```python
from build123d import *

# Parameters (mm, degrees)
F1_DEPTH = 10


with BuildPart() as f1:
    # F0 (on Top) → F1 (new body)
    with BuildSketch(Plane.XY):
        Polygon((2.178894, 24.904867), (0, 25), (0, 29.088151), (-5.051104, 28.646236), (-4.341204, 24.620194), (-6.470476, 24.148146), (-7.528567, 28.096996), (-12.293184, 26.362817), (-10.565457, 22.657695), (-12.5, 21.650635), (-14.544075, 25.191077), (-18.697503, 22.282816), (-16.06969, 19.151111), (-17.67767, 17.67767), (-20.568429, 20.568429), (-23.827618, 16.684278), (-20.478801, 14.339411), (-21.650635, 12.5), (-25.191077, 14.544075), (-27.333921, 9.948733), (-23.492316, 8.550504), (-24.148146, 6.470476), (-28.096996, 7.528567), (-28.977462, 2.535199), (-24.904867, 2.178894), (-25, 0), (-29.088151, 0), (-28.646236, -5.051104), (-24.620194, -4.341204), (-24.148146, -6.470476), (-28.096996, -7.528567), (-26.362817, -12.293184), (-22.657695, -10.565457), (-21.650635, -12.5), (-25.191077, -14.544075), (-22.282816, -18.697503), (-19.151111, -16.06969), (-17.67767, -17.67767), (-20.568429, -20.568429), (-16.684278, -23.827618), (-14.339411, -20.478801), (-12.5, -21.650635), (-14.544075, -25.191077), (-9.948733, -27.333921), (-8.550504, -23.492316), (-6.470476, -24.148146), (-7.528567, -28.096996), (-2.535199, -28.977462), (-2.178894, -24.904867), (0, -25), (0, -29.088151), (5.051104, -28.646236), (4.341204, -24.620194), (6.470476, -24.148146), (7.528567, -28.096996), (12.293184, -26.362817), (10.565457, -22.657695), (12.5, -21.650635), (14.544075, -25.191077), (18.697503, -22.282816), (16.06969, -19.151111), (17.67767, -17.67767), (20.568429, -20.568429), (23.827618, -16.684278), (20.478801, -14.339411), (21.650635, -12.5), (25.191077, -14.544075), (27.333921, -9.948733), (23.492316, -8.550504), (24.148146, -6.470476), (28.096996, -7.528567), (28.977462, -2.535199), (24.904867, -2.178894), (25, 0), (29.088151, 0), (28.646236, 5.051104), (24.620194, 4.341204), (24.148146, 6.470476), (28.096996, 7.528567), (26.362817, 12.293184), (22.657695, 10.565457), (21.650635, 12.5), (25.191077, 14.544075), (22.282816, 18.697503), (19.151111, 16.06969), (17.67767, 17.67767), (20.568429, 20.568429), (16.684278, 23.827618), (14.339411, 20.478801), (12.5, 21.650635), (14.544075, 25.191077), (9.948733, 27.333921), (8.550504, 23.492316), (6.470476, 24.148146), (7.528567, 28.096996), (2.535199, 28.977462), align=None)
    extrude(amount=F1_DEPTH)


solid = f1.part
```
The listing builds one solid part. Answer for the finished solid, in the listing's coordinates (mm). A direction names the side the tool comes from. Coordinates: 2 decimals unless noted, no trailing zeros. Loops run counter-clockwise (first coordinate to the right, second up) from the corner with the lowest first, then second, coordinate; pieces in that order, holes last. Notation, with made-up numbers: M 79,40 L 115,40 A26 ccw 115,64 Z; hole C 63,33 d9. An arc over 180 degrees is marked long. Answer as a JSON object with one key per item and string values. Group by question number.
Item 1: Each of these flat-tipped pins is pushed along its axis until it touches: P1, Ø2, axis at x = 27, z = 7.5, coming from the -Y side; P2, Ø4, axis at x = -5, z = 4, coming from the +Y side; P3, Ø5, axis at x = -4, z = 6.5, coming from the +Y side. Where does it stop, or does it pass through?
Item 2: Which of the six approach directions +Z, -Z, +X, -X, +Y, -Y give full straight-line access (tool end or side, diameter ignored) to faces 1 (the face through (-28.53, 5.07, 4.93)), 2 (the face through (0, 27, 5)), 3 (the face through (-1.1, -24.95, 4.93)), 4 (the face through (25.44, -9.26, 4.93)), 5 (the face through (6.99, 26.09, 4.93))?
Item 3: Determine the mould class of faces 6 (the face through (9.26, 25.44, 4.93)), 7 (the face through (24.95, -1.1, 4.93)), 8 (the face through (6.99, -26.09, 4.93)), 9 (the face through (5.391, -24.387, 4.93)) for opening direction Y: +Y half, -Y half, draft (parallel to the pull), parting line (faces both ways), or undercut.
Item 4: Section B-B (y = -11.5) is taken. Write down the section's boundary in (x, z), and give its area (3 significant figures).
Item 5: Section A-A (y = 13.5) is taken. Write down the section's boundary in (x, z), and give its area (3 significant figures).
Item 6: Consider L1, parallel to X at y = -18.5, z = 8.25; L2, parallel to X at y = 25.5, z = 4.25; L3, parallel to X at y = 26, z = 3.75. Determine where each line is inside the solid, lowest interval first.
Solved:
{
 "1": {"P1": "stops at y = -12.81", "P2": "stops at y = 28.83", "P3": "stops at y = 28.96"},
 "2": {"face 1": "+Z, -Z, -X, +Y", "face 2": "+Z, -Z, +Y", "face 3": "+Z, -Z, -Y", "face 4": "+Z, -Z, +X", "face 5": "+Z, -Z"},
 "3": {"face 6": "+Y half", "face 7": "undercut", "face 8": "-Y half", "face 9": "undercut"},
 "4": {"outline": "M -26.65,0 L -24.66,0 L -24.66,10 L -26.65,10 Z; M -22.17,0 L 26.61,0 L 26.61,10 L -22.17,10 Z", "area": "508 mm2"},
 "5": {"outline": "M -25.68,0 L -23.38,0 L -23.38,10 L -25.68,10 Z; M -21.01,0 L 23.38,0 L 23.38,10 L -21.01,10 Z", "area": "467 mm2"},
 "6": {"L1": "x = -22.42 to -22.05, -18.5 to 16.78, 18.5 to 22.3", "L2": "x = -11.89 to -6.83, -4.5 to 0, 2.23 to 6.83, 9.28 to 13.88", "L3": "x = -12.12 to -6.97, -4.58 to 0, 2.27 to 6.97, 9.46 to 12.81"}
}
